Build history of the part. All positions in model axes, mm. Give positions to 0.01 mm unless a question says otherwise; leave off trailing zeros. Loops run counter-clockwise (first coordinate to the right, second up) from the corner with the lowest first, then second, coordinate; pieces in that order, holes last. Notation, with made-up numbers: M 55.5,-23 L 93.5,-23 A14 ccw 93.5,-16 Z; hole C 57,66 d4. An arc over 180 degrees is marked long. Answer as a JSON object with one key per item and string values. Group by question number.
1. Drill centre lines: line 1 along X through (y, z) = (15.5, -138); line 2 along X through (y, z) = (1.5, -250.5); line 3 along Y through (x, z) = (-14.75, -91.5). Where is each one in solid material? Low to high. Write a range as [from, to].
2. Slice it at C-C (y = 13.5). List the corners of the cut face in (x, z).
3. Drop flat-ended pins along their axis: pin 1 Ø1 at (x, z) = (3, -77.5) entering from -Y; pin 2 Ø1.5 at (x, z) = (0, -151) entering from -Y; pin 3 Ø3 at (y, z) = (13, -206.5) entering from +X. Give the stop position or say it passes through.
4. Slice it at A-A (x = -13.75). List the corners of the cut face in (y, z).
5. Mould opens along X. For faces 1 (the face through (-7, 11, 0)), 2 (the face through (1.905, 24, -141)), 3 (the face through (-8.739, -0.364, -140.875)), 4 (the face through (-9.041, 0.894, -140.875)) say: released by +X, released by -X, zero draft, split by the parting line, or undercut.
from build123d import *

# Parameters (mm, degrees)
EXTRUDE_THIN1_DEPTH = 285.75
FILLET1_R           = 1.27


with BuildPart() as part:
    # Sketch1 → Extrude-Thin1 (new body)
    with BuildSketch(Plane.XY):
        with BuildLine():
            Line((0, 0), (-19.05, -0.79375))
            Line((-19.05, -0.79375), (-19.05, 4.7625))
            ThreePointArc((-19.05, 4.7625), (-9.824616787, 7.648549572), (-6.35, 16.66875))
            Line((-6.35, 16.66875), (-7.9375, 16.66875))
            Line((-7.9375, 16.66875), (-7.9375, 20.6375))
            Line((-7.9375, 20.6375), (-6.35, 20.6375))
            ThreePointArc((-6.35, 20.6375), (-5.539033157, 24.253773684), (-2.38125, 26.19375))
            Line((-2.38125, 26.19375), (-2.38125, 27.78125))
            Line((-2.38125, 27.78125), (3.175, 27.78125))
            Line((3.175, 27.78125), (3.175, 21.43125))
            Line((3.175, 21.43125), (1.905, 21.43125))
            Line((1.905, 21.43125), (1.905, 26.51125))
            Line((1.905, 26.51125), (-1.11125, 26.51125))
            Line((-1.11125, 26.51125), (-1.11125, 24.934167832))
            ThreePointArc((-1.11125, 24.934167832), (-4.660969167, 23.278250334), (-4.440513376, 19.3675))
            Line((-4.440513376, 19.3675), (-6.6675, 19.3675))
            Line((-6.6675, 19.3675), (-6.6675, 17.93875))
            Line((-6.6675, 17.93875), (-5.236398958, 17.93875))
            ThreePointArc((-5.236398958, 17.93875), (-8.043524077, 7.673709188), (-17.78, 3.378124142))
            Line((-17.78, 3.378124142), (-17.78, 0.530268619))
            Line((-17.78, 0.530268619), (-0.052870792, 1.268899003))
            Line((-0.052870792, 1.268899003), (0, 0))
        make_face()
    extrude(amount=-EXTRUDE_THIN1_DEPTH)

    # Fillet1
    fillet1_edges = [part.edges().sort_by_distance(p)[0] for p in [
        (-1.11125, 24.934167832, -142.875),
        (-4.440513376, 19.3675, -142.875),
        (-5.236398958, 17.93875, -142.875),
        (-19.05, -0.79375, -142.875),
        (-19.05, 4.7625, -142.875),
        (-7.9375, 16.66875, -142.875),
        (-7.9375, 20.6375, -142.875),
        (-2.38125, 27.78125, -142.875),
        (3.175, 27.78125, -142.875),
    ]]
    fillet(fillet1_edges, radius=FILLET1_R)


solid = part.part
Established:
{
 "1": {"line 1": "x = [-6.32, -5.05]", "line 2": "x = [-19.05, -17.78]", "line 3": "y = [-0.61, 0.66], [3.67, 4.97]"},
 "2": {"outline": "M -6.54,-285.75 L -5.25,-285.75 L -5.25,0 L -6.54,0 Z"},
 "3": {"pin 1": "stops at y = 21.43", "pin 2": "stops at y = -0.03", "pin 3": "stops at x = -5.11"},
 "4": {"outline": "M -0.57,-285.75 L 0.7,-285.75 L 0.7,0 L -0.57,0 Z; M 3.93,-285.75 L 5.27,-285.75 L 5.27,0 L 3.93,0 Z"},
 "5": {"face 1": "zero draft", "face 2": "undercut", "face 3": "released by +X", "face 4": "undercut"}
}
